Work out the finished part from the listing and answer in its coordinate system (mm). A direction names the side the tool comes from. Round coordinates to 2 decimals unless told otherwise and drop trailing zeros. Order: outer loops, then holes, each group sorted by start corner. A loop starts at its lowest first (then second) coordinate and runs counter-clockwise, first axis right, second up. Notation, with made-up numbers: (-2.5, 50) - (38.5, 50) arc R17 cw to (38.5, 74) - close; hole circle Ø3 at (-27.75, 21.25). An arc over 180 degrees is marked (long way). Use one line per item in the form item = value. Start each with the question number.
Q1. The part is cut by section B-B on y = 0. Determine the outline of the cut face in (x, z).
Q2. Given P1, Ø1.5, axis at y = 33, z = 1.5, coming from the -X side; P2, Ø10, axis at x = 24.5, y = -29, coming from the +Z side; P3, Ø0.6, axis at x = -39, z = 3.5, coming from the -Y side, each flat-ended and moving along its own axis, determine where each tip first touches the part or whether it passes through.
Q3. The part is cut by section A-A on z = 5.5. Determine the outline of the cut face in (x, y), plus the area to 3 significant figures.
Q4. Find the intervals of material crossed by line 1 (X direction, y = 0, z = 3); line 2 (X direction, y = -0.5, z = 11); line 3 (Y direction, x = -1, z = 9.25), in increasing order. Write a range as [from, to].
Q5. The part is cut by section D-D on x = 14. Determine the outline of the cut face in (y, z).
Q6. Which of the six approach directions +Z, -Z, +X, -X, +Y, -Y give full straight-line access (tool end or side, diameter ignored) to faces 1 (the flat face through (-28, 27, 2)), 2 (the flat face through (-10, 40, 3)), 3 (the cylindrical face through (-0.1, -38.3, 7.8))?
from build123d import *

# Parameters (mm, degrees)
SKETCH_R        = 45
SKETCH_R_2      = 37.5
PAD_DEPTH       = 2
SKETCH001_R     = 38.3
SKETCH001_R_2   = 37.5
PAD001_DEPTH    = 10
CHAMFER_SIZE    = 0.3
CHAMFER001_SIZE = 0.3
SKETCH002_W     = 38.775471
SKETCH002_H     = 41.534115
SKETCH002_W_2   = 92.953724
SKETCH002_H_2   = 53.076206
SKETCH002_W_3   = 93.597454
SKETCH002_H_3   = 43.392277
SKETCH002_W_4   = 61.284782
SKETCH002_H_4   = 58.713959
POCKET_DEPTH    = 10.001
PAD002_DEPTH    = 2


with BuildPart() as part:
    # Sketch → Pad (new body)
    with BuildSketch(Plane.XY):
        Circle(SKETCH_R)
        Circle(SKETCH_R_2, mode=Mode.SUBTRACT)
    extrude(amount=PAD_DEPTH)

    # Sketch001 (on Face4 of Pad) → Pad001 (join)
    with BuildSketch(Plane.XY.offset(2)):
        Circle(SKETCH001_R)
        Circle(SKETCH001_R_2, mode=Mode.SUBTRACT)
    extrude(amount=PAD001_DEPTH)

    # Chamfer
    chamfer_edges = [part.edges().sort_by_distance(p)[0] for p in [
        (-37.5, 0, 12),
    ]]
    chamfer(chamfer_edges, length=CHAMFER_SIZE)

    # Chamfer001
    chamfer001_edges = [part.edges().sort_by_distance(p)[0] for p in [
        (-38.3, 0, 12),
    ]]
    chamfer(chamfer001_edges, length=CHAMFER001_SIZE)

    # Sketch002 (on Face6 of Chamfer001) → Pocket (cut, through all)
    with BuildSketch(Plane.XY.offset(2)):
        with Locations((-29.387735, 30.767057)):
            Rectangle(SKETCH002_W, SKETCH002_H)
        with Locations((56.476862, 36.538103)):
            Rectangle(SKETCH002_W_2, SKETCH002_H_2)
        with Locations((56.798727, -31.696138)):
            Rectangle(SKETCH002_W_3, SKETCH002_H_3)
        with Locations((-40.642391, -39.35698)):
            Rectangle(SKETCH002_W_4, SKETCH002_H_4)
    extrude(amount=POCKET_DEPTH, mode=Mode.SUBTRACT)

    # Sketch003 (on Face31 of Pocket) → Pad002 (join)
    with BuildSketch(Plane.XY.offset(2)):
        with BuildLine():
            ThreePointArc((10, 43.874822), (0, 45), (-10, 43.874822))
            Line((-10, 36.142081), (-10, 43.874822))
            ThreePointArc((10, 36.142081), (0, 37.5), (-10, 36.142081))
            Line((10, 43.874822), (10, 36.142081))
        make_face()
        with BuildLine():
            Line((-10, -43.874822), (-10, -36.142081))
            ThreePointArc((-10, -36.142081), (0, -37.5), (10, -36.142081))
            Line((10, -36.142081), (10, -43.874822))
            ThreePointArc((-10, -43.874822), (0, -45), (10, -43.874822))
        make_face()
        with BuildLine():
            Line((-43.874822, 10), (-36.142081, 10))
            ThreePointArc((-36.142081, 10), (-37.5, 0), (-36.142081, -10))
            Line((-36.142081, -10), (-43.874822, -10))
            ThreePointArc((-43.874822, 10), (-45, 0), (-43.874822, -10))
        make_face()
        with BuildLine():
            Line((43.874822, -10), (36.142081, -10))
            ThreePointArc((36.142081, -10), (37.5, 0), (36.142081, 10))
            Line((36.142081, 10), (43.874822, 10))
            ThreePointArc((43.874822, -10), (45, 0), (43.874822, 10))
        make_face()
    extrude(amount=PAD002_DEPTH)


solid = part.part
Found:
q1.outline = (-45, 0) - (-37.5, 0) - (-37.5, 11.7) - (-37.8, 12) - (-38, 12) - (-38.3, 11.7) - (-38.3, 4) - (-45, 4) - close; (37.5, 0) - (45, 0) - (45, 4) - (38.3, 4) - (38.3, 11.7) - (38, 12) - (37.8, 12) - (37.5, 11.7) - close
q2.P1 = -31.38
q2.P2 = 2
q2.P3 = -10
q3.outline = (-36.97, -10) - (-36.14, -10) arc R37.5 cw to (-36.14, 10) - (-36.97, 10) arc R38.3 ccw to start; (-10, -36.97) arc R38.3 ccw to (10, -36.97) - (10, -36.14) arc R37.5 cw to (-10, -36.14) - close; (-10, 36.14) arc R37.5 cw to (10, 36.14) - (10, 36.97) arc R38.3 ccw to (-10, 36.97) - close; (36.14, -10) - (36.97, -10) arc R38.3 ccw to (36.97, 10) - (36.14, 10) arc R37.5 cw to start
q3.area = 64.8 mm²
q4.line_1 = [-45, -37.5], [37.5, 45]
q4.line_2 = [-38.3, -37.5], [37.5, 38.3]
q4.line_3 = [-38.29, -37.49], [37.49, 38.29]
q5.outline = (-42.77, 0) - (-34.79, 0) - (-34.79, 2) - (-42.77, 2) - close; (34.79, 0) - (42.77, 0) - (42.77, 2) - (34.79, 2) - close
q6.face_1 = +Z, -X, +Y
q6.face_2 = +Z, -X, +Y, -Y
q6.face_3 = +Z, -Y
